Part model, mm, in its own coordinate system. A direction names the side the tool comes from. Coordinates: 2 decimals unless noted, no trailing zeros. Write each loop counter-clockwise with the first axis right and the second up, starting at its lowest first coordinate (ties: lowest second). Pieces come first, ordered by that corner, then holes. Notation, with made-up numbers: (-19, 20) - (0, 20) arc R14 ccw to (0, 44) - close; hole circle Ø3 at (30.25, -32). An arc over 180 degrees is marked (long way). Write each question's results on one line, items separated by ' | '.
from build123d import *

# Parameters (mm, degrees)
SKETCH1_R           = 70
SKETCH1_R_2         = 30
BOSS_EXTRUDE1_DEPTH = 40
SKETCH2_R           = 75
SKETCH2_R_2         = 30
BOSS_EXTRUDE2_DEPTH = 10
CUT_EXTRUDE1_DEPTH  = 146.773797371


with BuildPart() as part:
    # Sketch1 → Boss-Extrude1 (new, symmetric)
    with BuildSketch(Plane(origin=(0, 0, 0), x_dir=(1, 0, 0), z_dir=(0, 1, 0))):
        with Locations(Location((0, 0, 0), (0, 0, 270))):
            Circle(SKETCH1_R)
        with Locations(Location((0, 0, 0), (0, 0, 270))):
            Circle(SKETCH1_R_2, mode=Mode.SUBTRACT)
    extrude(amount=BOSS_EXTRUDE1_DEPTH, both=True)

    # Sketch2 → Boss-Extrude2 (add)
    with BuildSketch(Plane(origin=(0, 40, 0), x_dir=(1, 0, 0), z_dir=(0, 1, 0))):
        with Locations(Location((0, 0, 0), (0, 0, 270))):
            Circle(SKETCH2_R)
        with Locations(Location((0, 0, 0), (0, 0, 270))):
            Circle(SKETCH2_R_2, mode=Mode.SUBTRACT)
    boss_extrude2 = extrude(amount=BOSS_EXTRUDE2_DEPTH)

    # Mirror1: Boss-Extrude2 across plane
    add(boss_extrude2.mirror(Plane.ZX))

    # Sketch3 → Cut-Extrude1 (cut, through all)
    with BuildSketch(Plane.XZ.offset(50)):
        with BuildLine():
            Line((-9, 33.20180718), (-9, 19.467949782))
            Line((-9, 19.467949782), (9, 19.467949782))
            Line((9, 19.467949782), (9, 33.20180718))
            ThreePointArc((9, 33.20180718), (0, 34.4), (-9, 33.20180718))
        make_face()
    extrude(amount=-CUT_EXTRUDE1_DEPTH, mode=Mode.SUBTRACT)


solid = part.part
(1) 3-axis set-ups, long thin cutter, end or side, ignore diameter. For faces 1 (the flat face through (-32, -50, -1)), 2 (the cylindrical face through (0.1, -0.7, 34.4)), 3 (the cylindrical face through (-42.594, 0.56, -55.55)): which of +Z, -Z, +X, -X, +Y, -Y reach the whole face in a straight line?
Return value:
face 1: +Z, -Z, +X, -X, -Y | face 2: +Y, -Y | face 3: none
(2) Flat gauge pins, fed straight in: P1, Ø4, axis at y = 14, z = 44.5, coming from the +X side; P2, Ø1, axis at y = 16, z = -7, coming from the +X side; P3, Ø10, axis at y = 34, z = -3, coming from the -X side. Where does each tip first touch, or does it go through?
Return value:
P1: stops at x = 55.62 | P2: stops at x = 69.7 | P3: stops at x = -70
(3) Saw through at B-B on x = 0. Write the cut outline in (y, z).
Return value:
outline: (-50, -75) - (-40, -75) - (-40, -70) - (40, -70) - (40, -75) - (50, -75) - (50, -30) - (-50, -30) - close; (-50, 34.4) - (50, 34.4) - (50, 75) - (40, 75) - (40, 70) - (-40, 70) - (-40, 75) - (-50, 75) - close
(4) Saw through at C-C on y = 16.5. Write the cut outline in (x, z), then the cut area to 3 significant figures.
Return value:
outline: circle Ø140 at (0, 0); hole (-9, 28.62) arc R30 ccw (long way) to (9, 28.62) - (9, 33.2) arc R34.4 ccw to (-9, 33.2) - close | area: 12,500 mm^2
(5) Saw through at D-D on x = -44.5. Write the cut outline in (y, z), then the cut area to 3 significant figures.
Return value:
outline: (-50, -60.37) - (-40, -60.37) - (-40, -54.03) - (40, -54.03) - (40, -60.37) - (50, -60.37) - (50, 60.37) - (40, 60.37) - (40, 54.03) - (-40, 54.03) - (-40, 60.37) - (-50, 60.37) - close | area: 11,100 mm^2
(6) Two-plate mould, pull along Y, no slides. Class faces 4 (the flat face through (-50, -40, 50)), 5 (the flat face through (-50, 40, 50)), 6 (the cylindrical face through (1.191, 0.7, -29.976)), 7 (the flat face through (-32, 50, -1)): released by +Y, released by -Y, zero draft, split by the parting line, or undercut.
Return value:
face 4: undercut | face 5: undercut | face 6: zero draft | face 7: released by +Y
(7) Saw through at A-A on z = 0. Write the cut outline in (x, y), then the cut area to 3 significant figures.
Return value:
outline: (-75, -50) - (-30, -50) - (-30, 50) - (-75, 50) - (-75, 40) - (-70, 40) - (-70, -40) - (-75, -40) - close; (30, -50) - (75, -50) - (75, -40) - (70, -40) - (70, 40) - (75, 40) - (75, 50) - (30, 50) - close | area: 8,200 mm^2
(8) Wall check: line 1 (X direction, y = -12.5, z = 0); line 2 (Y direction, x = -51, z = -48); line 3 (Z direction, x = -22, y = 14). Give the ranges that are in metal, low to high. Write a range as from..to.
Return value:
line 1: x = -70..-30, 30..70 | line 2: y = -50..-40, 40..50 | line 3: z = -66.45..-20.4, 20.4..66.45
